Could you check a few things on this model? Use its own coordinates, in mm. A direction names the side the tool comes from. Round coordinates to 2 decimals unless told otherwise and drop trailing zeros. Loops run counter-clockwise (first coordinate to the right, second up) from the corner with the lowest first, then second, coordinate; pieces in that order, holes last.
from build123d import *

# Parameters (mm, degrees)
SKETCH008_R        = 5
PAD003_DEPTH       = 30
SKETCH009_W        = 12
SKETCH009_H        = 21.7
POCKET002_DEPTH    = 20
SKETCH010_R        = 60
SKETCH010_R_2      = 6
PAD004_DEPTH       = 5
FILLET_R           = 4
BODY004_ROLL_ANGLE = 90


with BuildPart() as part:
    # Sketch008 → Pad003 (new body)
    with BuildSketch(Plane.YZ):
        with BuildLine():
            ThreePointArc((0, -18.042356), (18.042356, 0), (0, 18.042356))
            Line((0, 18.042356), (-5.957898, 18.042356))
            Line((-5.957898, -18.042356), (-5.957898, 18.042356))
            Line((0, -18.042356), (-5.957898, -18.042356))
        make_face()
        with Locations((10, 0)):
            Circle(SKETCH008_R, mode=Mode.SUBTRACT)
    extrude(amount=PAD003_DEPTH)

    # Sketch009 → Pocket002 (cut, symmetric)
    with BuildSketch(Plane.XY):
        with Locations((15, 10.85)):
            Rectangle(SKETCH009_W, SKETCH009_H)
    extrude(amount=POCKET002_DEPTH, both=True, mode=Mode.SUBTRACT)

    # Sketch010 → Pad004 (join)
    with BuildSketch(Plane(origin=(12, -3, 0), x_dir=(1, 0, 0), z_dir=(0, -1, 0))):
        Circle(SKETCH010_R)
        with Locations((0.190896, 37.924703)):
            Circle(SKETCH010_R_2, mode=Mode.SUBTRACT)
        with Locations((-36, -22.55)):
            Circle(SKETCH010_R_2, mode=Mode.SUBTRACT)
        with Locations((40, -8.84)):
            Circle(SKETCH010_R_2, mode=Mode.SUBTRACT)
    extrude(amount=PAD004_DEPTH)

    # Fillet
    fillet_edges = [part.edges().sort_by_distance(p)[0] for p in [
        (-48, -3, 0),
    ]]
    fillet(fillet_edges, radius=FILLET_R)


with BuildPart() as part_1:
    # Body004 roll: moved
    add(part.part.rotate(Axis((0, 0, 0), (1, 0, 0)), BODY004_ROLL_ANGLE))


with BuildPart() as part_2:
    # Body004 placement: moved
    add(part_1.part.moved(Location((0, 0, 21))))


solid = part_2.part
Item 1: Will these pins go through, and if not, where does the flat tip stop? pin 1 (3.5 mm diameter, centred on x = 14, y = 2, fed in from +Z); pin 2 (14 mm diameter, centred on x = 12.19, y = -37.92, fed in from +Z); pin 3 (5.5 mm diameter, centred on y = 4.5, z = 33.5, fed in from +X); pin 4 (1.5 mm diameter, centred on y = -20, z = 20, fed in from -X).
Results list:
pin 1: stops at z = 21
pin 2: stops at z = 18
pin 3: stops at x = 30
pin 4: passes through
Item 2: For faces 1 (the flat face through (15, 18.042, 20)), 2 (the flat face through (0, 0, 24)), 3 (the flat face through (30, 0, 24)), 4 (the flat face through (9, -4.3, 27.9)), which set-ups out of +Z, -Z, +X, -X, +Y, -Y let a thin tool reach every point of the face, with its end or its side?
Results list:
face 1: +Z, +X, -X, +Y
face 2: +Z, -X, +Y, -Y
face 3: +Z, +X, +Y, -Y
face 4: +Z, +Y, -Y
Item 3: We'd pull the mould along Z, two halves only. Please class faces 5 (the flat face through (15, -18.042, 20)), 6 (the flat face through (15, 0, 21)), 7 (the cylindrical face through (25, 0, 26)): released by +Z, released by -Z, zero draft, split by the parting line, or undercut.
Results list:
face 5: zero draft
face 6: released by +Z
face 7: undercut
Item 4: If we section it at A-A, the plane y = 0: Please give me the cut outline in (x, z), then the cut area to 3 significant figures.
Results list:
outline: (-48, 13) - (72, 13) - (72, 14) arc R4 ccw to (68, 18) - (30, 18) - (30, 26) - (21, 26) - (21, 21) - (9, 21) - (9, 26) - (0, 26) - (0, 18) - (-44, 18) arc R4 ccw to (-48, 14) - close; (0, 36) - (9, 36) - (9, 39.04) - (0, 39.04) - close; (21, 36) - (30, 36) - (30, 39.04) - (21, 39.04) - close
area: 828 mm2
Item 5: If I drill on line 1 along Z through (x, y) = (10.5, -18); line 2 along Y through (x, z) = (4, 29); line 3 along Z through (x, y) = (61.5, -10), over which ranges is the centre line in solid material (lowest first)?
Results list:
line 1: z = 13 to 21
line 2: y = -16.17 to -4.58, 4.58 to 16.17
line 3: z = 13 to 18
Item 6: If we section it at B-B, the plane z = 28: Please give me the cut outline in (x, y), then the cut area to 3 significant figures.
Results list:
outline: (0, -16.63) - (9, -16.63) - (9, -4) - (0, -4) - close; (0, 4) - (9, 4) - (9, 16.63) - (0, 16.63) - close; (21, -16.63) - (30, -16.63) - (30, -4) - (21, -4) - close; (21, 4) - (30, 4) - (30, 16.63) - (21, 16.63) - close
area: 455 mm2
